Answer from the drawing. Dimensions are ordinates in mm from the lowest x, y and z of the part. A direction names the side the tool comes from. Round coordinates to 2 decimals unless told otherwise and drop trailing zeros. Loops run counter-clockwise (first coordinate to the right, second up) from the corner with the lowest first, then second, coordinate; pieces in that order, holes last. Notation, with made-up numbers: (68, -32) -> (102, -32) arc R16 cw to (102, -26) -> close; hole circle Ø10 at (73.25, -9). An arc over 180 degrees is marked (long way). One line per question, with ' | ' between items.
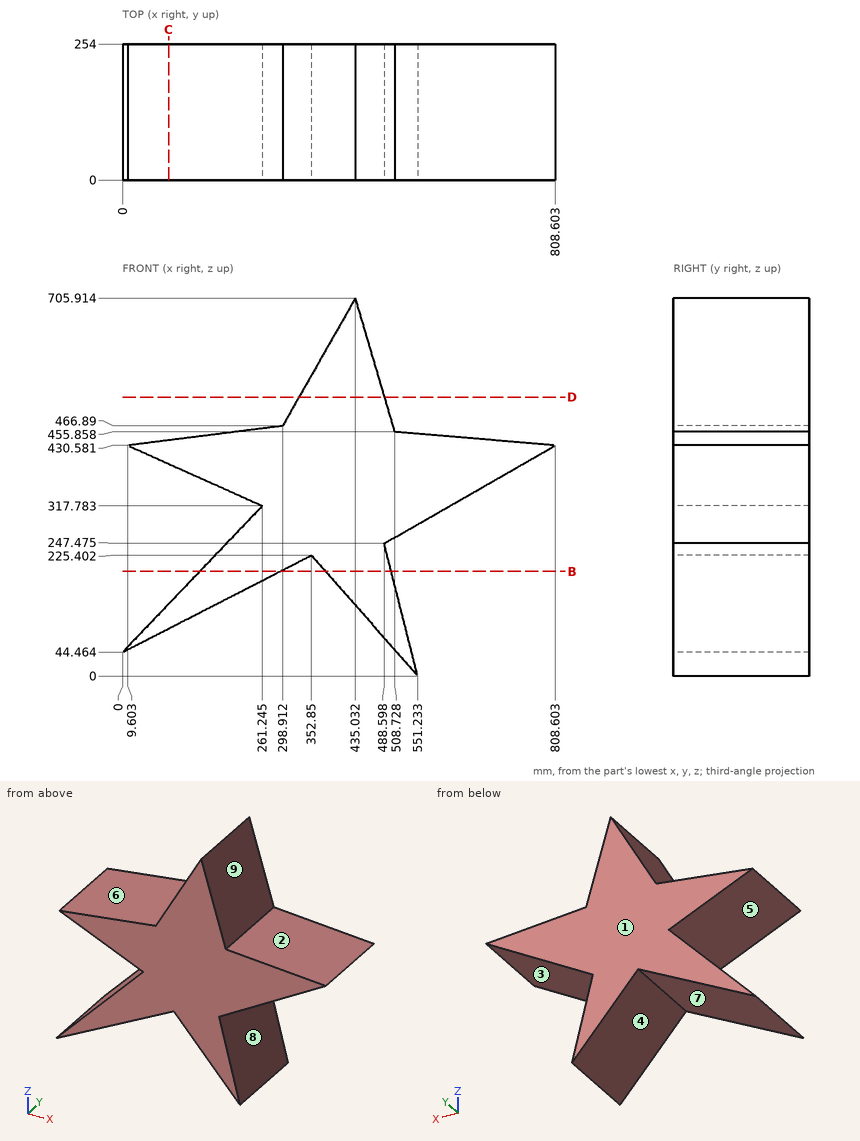
Q1. A cutting plane is placed at D-D on z = 521. Give the vertices of the cut face in (x, y).
Numbers:
outline: (329.73, 0) -> (489.53, 0) -> (489.53, 254) -> (329.73, 254) -> close
Q2. A cutting plane is placed at B-B on z = 195.5. Give the vertices of the cut face in (x, y), plus the area to 3 significant figures.
Numbers:
outline: (144.36, 0) -> (294.54, 0) -> (294.54, 254) -> (144.36, 254) -> close; (379.17, 0) -> (501.75, 0) -> (501.75, 254) -> (379.17, 254) -> close | area: 69,300 mm^2
Q3. For a pull along Z with two mould halves and no side action, classify the marked faces 1, 2, 3 and 4 as pulls with the +Z half, pulls with the -Z half, needs draft (parallel to the pull), parting line crosses it, or undercut.
Numbers:
face 1: needs draft | face 2: pulls with the +Z half | face 3: undercut | face 4: pulls with the -Z half
Q4. Given pin 1 Ø6 at (x, y) = (266.5, 66) entering from +Z; pin 2 Ø10 at (x, y) = (711.5, 100) entering from -Z; pin 3 Ø8 at (y, z) = (174, 601) entering from -X, each flat-ended and moving along its own axis, determine where each tip first touches the part or whether it passes through.
Numbers:
pin 1: z = 463.2 | pin 2: z = 372.16 | pin 3: x = 373.01
Q5. Find the intervals of material crossed by line 1 (Z direction, x = 113, y = 148) (1 decimal); line 2 (Z direction, x = 236, y = 63) (1 decimal); line 3 (Z direction, x = 331, y = 128) (1 decimal), in increasing order. Write a range as from..to.
Numbers:
line 1: 102.4..162.7, 384.2..443.6 | line 2: 165.5..291.4, 329.1..459 | line 3: 214.2..523.2
Q6. A cutting plane is placed at C-C on x = 86. Give the vertices of the cut face in (y, z), plus the area to 3 significant figures.
Numbers:
outline: (0, 88.56) -> (254, 88.56) -> (254, 134.44) -> (0, 134.44) -> close; (0, 396.34) -> (254, 396.34) -> (254, 440.17) -> (0, 440.17) -> close | area: 22,800 mm^2
Q7. For the marked faces 5, 6, 7, 8 and 9, determine the directions among +Z, -Z, +X, -X, +Y, -Y from which every point of the face is accessible in a straight line to the end or side of a thin tool.
Numbers:
face 5: -X, +Y, -Y | face 6: +Z, -X, +Y, -Y | face 7: -Z, +Y, -Y | face 8: +X, +Y, -Y | face 9: +Z, +X, +Y, -Y
